CAD build for the part. Positions are in the model's coordinates, mm. A direction names the side the tool comes from. Give positions to 0.01 mm unless a question says otherwise; leave off trailing zeros. Loops run counter-clockwise (first coordinate to the right, second up) from the corner with the lowest first, then second, coordinate; pieces in that order, holes last. Notation, with made-up numbers: M 49,-17.5 L 67,-17.5 A22 cw 67,13.5 Z; hole C -18.5,67 d11. An arc over 180 degrees is marked long. Answer as CSV lines item,"result".
Autodesk Inventor part; units mm, degrees
ref_plane "Work Plane2" through (-89, -40.3889, 33.5) normal (0, 0, 1) x (1, 0, 0)
ref_plane "YZ Plane" through (0, 0, 0) normal (1, 0, 0) x (0, 1, 0)
ref_plane "XZ Plane" through (0, 0, 0) normal (0, 1, 0) x (-1, 0, 0)
ref_plane "Work Plane1" through (0, 0, 0) normal (0, 0, 1) x (1, 0, 0)
ref_plane "Work Plane2" through (-89, -40.3889, 33.5) normal (0, 0, 1) x (1, 0, 0)
sketch "Sketch1" plane through (0, 0, 0) normal (0, 0, 1) x (1, 0, 0)
  line L0 (23.5, 88.5) -> (-23.5, 88.5)
  line L1 (-23.5, 88.5) -> (-23.5, 36.5)
  line L2 (-26.5, 33.5) -> (-89, 33.5)
  line L3 (-89, 33.5) -> (-89, -72.5)
  line L4 (-89, -72.5) -> (-77, -72.5)
  line L5 (-74, -75.5) -> (-74, -93.5)
  line L6 (-74, -93.5) -> (74, -93.5)
  line L7 (74, -93.5) -> (74, -75.5)
  line L8 (77, -72.5) -> (89, -72.5)
  line L9 (89, -72.5) -> (89, 33.5)
  line L10 (89, 33.5) -> (26.5, 33.5)
  line L11 (23.5, 36.5) -> (23.5, 88.5)
  line L12 (-4.5, 81.5) -> (-4.5, 36.5)
  line L13 (-7.5, 33.5) -> (-13.5, 33.5)
  line L14 (-16.5, 36.5) -> (-16.5, 81.5)
  line L15 (-13.5, 84.5) -> (-7.5, 84.5)
  line L16 (16.5, 81.5) -> (16.5, 36.5)
  line L17 (13.5, 33.5) -> (7.5, 33.5)
  line L18 (4.5, 36.5) -> (4.5, 81.5)
  line L19 (7.5, 84.5) -> (13.5, 84.5)
  line L20 (-4.5, 88.5) -> (4.5, 88.5)
  line L21 (4.5, 88.5) -> (4.5, 3.75)
  line L22 (4.5, 3.75) -> (-4.5, 3.75)
  line L23 (-4.5, 3.75) -> (-4.5, 88.5)
  line L24 (-32.2, 4.75) -> (-59.9, 4.75)
  arc A0 (13.5, 33.5) -> (16.5, 36.5) centre (13.5, 36.5) ccw
  arc A1 (4.5, 36.5) -> (7.5, 33.5) centre (7.5, 36.5) ccw
  arc A2 (7.5, 84.5) -> (4.5, 81.5) centre (7.5, 81.5) ccw
  arc A3 (16.5, 81.5) -> (13.5, 84.5) centre (13.5, 81.5) ccw
  arc A4 (-4.5, 81.5) -> (-7.5, 84.5) centre (-7.5, 81.5) ccw
  arc A5 (-7.5, 33.5) -> (-4.5, 36.5) centre (-7.5, 36.5) ccw
  arc A6 (-16.5, 36.5) -> (-13.5, 33.5) centre (-13.5, 36.5) ccw
  arc A7 (-13.5, 84.5) -> (-16.5, 81.5) centre (-13.5, 81.5) ccw
  arc A8 (-26.5, 33.5) -> (-23.5, 36.5) centre (-26.5, 36.5) ccw
  arc A9 (-74, -75.5) -> (-77, -72.5) centre (-77, -75.5) ccw
  arc A10 (77, -72.5) -> (74, -75.5) centre (77, -75.5) ccw
  arc A11 (23.5, 36.5) -> (26.5, 33.5) centre (26.5, 36.5) ccw
  point P0 (0, 0)
  point P1 (-4.5, 81.5)
  point P2 (-4.5, 36.5)
  dimension "d0" = 1
extrude "Extrusion1" add sketch "Sketch1" along normal up to surface (33.5 mm away) contours L21 L18 L22 L23 L12 L0
sketch "Sketch2" plane through (4.5, 3.75, 0) normal (1, 0, 0) x (0, 0, -1)
  circle A0 centre (-23.4363, 30.1825) radius 2
  point P0 (0, -3.75)
extrude "Extrusion2" cut sketch "Sketch2" against normal blind 10
sketch "Sketch3" plane through (4.5, 3.75, 0) normal (1, 0, 0) x (0, 0, -1)
  circle A0 centre (-10.5, 57.25) radius 4.5
  point P0 (0, -3.75)
extrude "Extrusion3" cut sketch "Sketch3" against normal blind 4
sketch "Sketch4" plane through (-4.5, 3.75, 0) normal (-1, 0, 0) x (0, 0, 1)
  circle A0 centre (10.5, 57.25) radius 4.5
  point P0 (0, -3.75)
extrude "Extrusion4" cut sketch "Sketch4" against normal blind 4
sketch "Sketch5" plane through (-4.5, 3.75, 33.5) normal (0, 0, 1) x (1, 0, 0)
  line L0 (5, 61.75) -> (5, 52.75)
  line L1 (4, 52.75) -> (4, 61.75)
  line L2 (9, 28.1825) -> (0, 28.1825)
  line L3 (9, 32.1825) -> (0, 32.1825)
  line L4 (17, 78.15) -> (-8, 78.15)
  line L5 (-8, 35.85) -> (17, 35.85)
  line L6 (9, 84.75) -> (9, 0)
  line L7 (0, 52.75) -> (0, 61.75)
  line L8 (9, 35.85) -> (0, 35.85)
  line L9 (0, 35.85) -> (0, 52.75)
  line L10 (0, 52.75) -> (9, 52.75)
  line L11 (9, 52.75) -> (9, 35.85)
  line L12 (0, 0) -> (0, 84.75)
  line L13 (9, 78.15) -> (0, 78.15)
  line L14 (0, 78.15) -> (0, 61.75)
  line L15 (0, 61.75) -> (9, 61.75)
  line L16 (9, 61.75) -> (9, 78.15)
  line L17 (-18, 8.625) -> (-18, 22.125)
  line L18 (-18, 15.375) -> (27, 15.375)
  line L19 (9, 35.85) -> (0, 52.75)
  line L20 (9, 61.75) -> (9, 52.75)
  line L21 (0, 35.85) -> (9, 52.75)
  line L22 (9, 61.75) -> (0, 78.15)
  line L23 (0, 61.75) -> (9, 78.15)
  point P0 (4.5, -3.75)
  point P1 (4.5, 15.375)
  point P2 (4.5, 44.3)
  point P3 (4.5, 69.95)
  dimension "d9" = 4.5
  dimension "d10" = 4.5
hole "Hole1" at (0, 19.125, 33.5) at (0, 48.05, 33.5) at (0, 73.7, 33.5) direction (0, 0, -1) diameter 3.6 end through all countersink diameter 6.6 countersink angle 90
sketch "Sketch6" plane through (-4.5, 3.75, 0) normal (0, -1, 0) x (1, 0, 0)
  line L0 (9, 33.5) -> (0, 33.5)
  line L1 (0, 0) -> (0, 33.5)
  line L2 (0, 0) -> (9, 0)
  line L3 (9, 0) -> (9, 33.5)
  line L4 (0, 16.75) -> (9, 16.75)
  line L5 (9, 16.75) -> (0, 33.5)
  line L6 (9, 33.5) -> (0, 16.75)
  line L7 (0, 16.75) -> (9, 0)
  line L8 (9, 16.75) -> (0, 0)
  point P0 (4.5, 0)
  point P1 (4.5, 8.375)
  point P2 (4.5, 25.125)
hole "Hole2" at (0, 3.75, 8.375) at (0, 3.75, 25.125) direction (0, 1, 0) diameter 4 depth 5.35 counterbore diameter 4.6 counterbore depth 0.75
sketch "Sketch7" plane through (-4.5, 88.5, 0) normal (0, 1, 0) x (1, 0, 0)
  line L0 (0, -33.5) -> (9, -33.5)
  line L1 (0, -33.5) -> (9, -33.5)
  line L2 (9, 0) -> (9, -33.5)
  line L3 (9, 0) -> (0, 0)
  line L4 (0, 0) -> (0, -33.5)
  line L5 (-8, -1.4) -> (-8, -6.6)
  line L6 (-8, -32.1) -> (-8, -26.9)
  line L7 (17, -32.1) -> (17, -26.9)
  line L8 (17, -1.4) -> (17, -6.6)
  line L9 (17, -32.1) -> (-8, -32.1)
  line L10 (-8, -32.1) -> (-8, -26.9)
  line L11 (-8, -26.9) -> (17, -26.9)
  line L12 (17, -26.9) -> (17, -32.1)
  line L13 (-8, -6.6) -> (17, -6.6)
  line L14 (17, -6.6) -> (17, -1.4)
  line L15 (17, -1.4) -> (-8, -1.4)
  line L16 (-8, -1.4) -> (-8, -6.6)
  line L17 (17, -6.6) -> (-8, -6.6)
  line L18 (-8, -6.6) -> (-8, -8.6)
  line L19 (-8, -8.6) -> (17, -8.6)
  line L20 (17, -8.6) -> (17, -6.6)
  line L21 (-8, -26.9) -> (17, -26.9)
  line L22 (17, -26.9) -> (17, -24.9)
  line L23 (17, -24.9) -> (-8, -24.9)
  line L24 (-8, -24.9) -> (-8, -26.9)
  line L25 (9, 0) -> (9, -33.5)
  line L26 (9, -16.75) -> (0, -16.75)
  line L27 (0, 0) -> (0, -33.5)
  line L28 (9, -24.9) -> (0, -16.75)
  line L29 (9, -8.6) -> (0, -16.75)
  line L30 (0, -8.6) -> (9, -16.75)
  line L31 (9, -16.75) -> (0, -24.9)
  point P0 (4.5, 0)
  point P1 (4.5, -20.825)
  point P2 (4.5, -12.675)
  dimension "d25" = 2
  dimension "d26" = 2
hole "Hole3" at (0, 88.5, 20.825) at (0, 88.5, 12.675) direction (0, -1, 0) diameter 4 depth 6.5 counterbore diameter 4.6 counterbore depth 2
sketch "Sketch8" plane through (-4.5, 3.75, 33.5) normal (0, 0, 1) x (1, 0, 0)
  line L0 (26, 27.2497) -> (-17, 27.2497)
  line L1 (26, 31.2497) -> (-17, 31.2497)
  line L2 (4, 52.75) -> (-1, 52.75)
  line L3 (4, 61.75) -> (-1, 61.75)
  line L4 (10, 61.75) -> (5, 61.75)
  line L5 (9, 52.75) -> (5, 52.75)
  line L6 (0, 0) -> (0, 84.75)
  line L7 (9, 52.75) -> (0, 52.75)
  line L8 (0, 52.75) -> (0, 61.75)
  line L9 (0, 61.75) -> (9, 61.75)
  line L10 (9, 61.75) -> (9, 52.75)
  line L11 (9, 28.1825) -> (0, 28.1825)
  line L12 (0, 31.2497) -> (9, 31.2497)
  line L13 (9, 31.2497) -> (9, 28.1825)
  line L14 (9, 28.1825) -> (0, 28.1825)
  line L15 (0, 28.1825) -> (0, 31.2497)
  line L16 (9, 28.1825) -> (0, 31.2497)
  line L17 (0, 28.1825) -> (9, 31.2497)
  line L18 (9, 52.75) -> (0, 61.75)
  line L19 (0, 52.75) -> (9, 61.75)
  point P0 (4.5, -3.75)
  point P1 (4.5, 29.7161)
  point P2 (4.5, 57.25)
hole "Hole4" at (0, 33.4661, 33.5) at (0, 61, 33.5) direction (0, 0, -1) diameter 4 depth 6 counterbore diameter 4.6 counterbore depth 1.5
properties part number "middle_gear_holder"
1) Which spindle directions (+Z, -Z, +X, -X, +Y, -Y) get a long thin tool onto all of the face, cutting with end or side? Do faces 1 (the face through (-0.5, 61, 10)), 2 (the face through (-0.088, 6.832, 27.123)), 3 (the face through (0, 82, 13)), 4 (the face through (0.689, 72.037, 15.776)), 5 (the face through (0, 63, 30)). Say none if no direction does.
Answer below:
face 1,"-X"
face 2,"-Y"
face 3,"+Y"
face 4,"+Z, -Z"
face 5,"+Z"
2) Mould opens along Z. For faces 6 (the face through (-4, 47, 33.5)), 7 (the face through (-0.54, 17.41, 15.78)), 8 (the face through (0.77, 84.22, 22.67)) say: +Z half, -Z half, draft (parallel to the pull), parting line (faces both ways), or undercut.
Answer below:
face 6,"+Z half"
face 7,"draft"
face 8,"undercut"
3) Band-saw the part on B-B on y = 61. Give the cut face in (x, z), and give its area (3 significant figures).
Answer below:
outline,"M -4.5,0 L 4.5,0 L 4.5,6 L 0.5,6 L 0.5,15 L 4.5,15 L 4.5,33.5 L 2.3,33.5 L 2.3,32 L 2,32 L 2,27.5 L -2,27.5 L -2,32 L -2.3,32 L -2.3,33.5 L -4.5,33.5 L -4.5,15 L -0.5,15 L -0.5,6 L -4.5,6 Z"
area,"205 mm^2"
4) Band-saw the part on A-A on y = 48.05. Give the cut face in (x, z), and give its area (3 significant figures).
Answer below:
outline,"M -4.5,0 L -1.8,0 L -1.8,32 L -3.3,33.5 L -4.5,33.5 Z; M 1.8,0 L 4.5,0 L 4.5,33.5 L 3.3,33.5 L 1.8,32 Z"
area,"179 mm^2"
5) Drill centre lines: line 1 (Y direction, x = -0.25, z = 16.5); line 2 (Z direction, x = 0, y = 87.25) (3 decimals); line 3 (Z direction, x = 0, y = 84.55) (3 decimals). Where is each one in solid material? Low to high. Write a range as from..to.
Answer below:
line 1,"y = 3.75..17.34, 20.91..46.27, 49.83..71.92, 75.48..88.5"
line 2,"z = 0..10.375, 14.975..18.525, 23.125..33.5"
line 3,"z = 0..10.675, 14.675..18.825, 22.825..33.5"
6) Flat gauge pins, fed straight in: pin 1 (1.2 mm diameter, centred on x = -0.5, z = 12, fed in from +Y); pin 2 (2.5 mm diameter, centred on x = -0.5, z = 25, fed in from -Y); pin 3 (2 mm diameter, centred on x = 0, y = 34, fed in from +Z). Where does each tip first touch, or does it go through?
Answer below:
pin 1,"stops at y = 82"
pin 2,"stops at y = 9.1"
pin 3,"stops at z = 27.5"
